Check sheet for the modelled part. Datum: model origin and axes. Units: mm. A direction names the side the tool comes from. Give positions to 0.01 mm unless a question says otherwise; leave off trailing zeros. Order: outer loops, then holes, each group sorted by start corner. A loop starts at its lowest first (then second) coordinate and runs counter-clockwise, first axis right, second up. Notation, with made-up numbers: (-5.5, 10.5) - (19.5, 10.5) arc R22 ccw to (19.5, 17.5) - close; hole circle Ø1 at (72, 24.25). An arc over 180 degrees is marked (long way). Answer in a Markdown table with one row per item.
from build123d import *

# Parameters (mm, degrees)
SKETCH1_R           = 10.5
BOSS_EXTRUDE1_DEPTH = 42
SKETCH3_R           = 14
BOSS_EXTRUDE2_DEPTH = 243
SKETCH4_R           = 9
BOSS_EXTRUDE3_DEPTH = 5
SKETCH5_W           = 36.2
SKETCH5_H           = 36.2
BOSS_EXTRUDE4_DEPTH = 35
BOSS_EXTRUDE4_TAPER = 5.710593137
SKETCH6_R           = 8
BOSS_EXTRUDE6_DEPTH = 3
SKETCH7_R           = 12
BOSS_EXTRUDE7_DEPTH = 25
CHAMFER1_SIZE       = 2
FILLET2_R           = 2.5
SKETCH8_W           = 3.5
SKETCH8_H           = 10
CHAMFER2_SIZE       = 2
CHAMFER3_SIZE       = 1
FILLET3_R           = 1.5


with BuildPart() as part:
    # Sketch1 → Boss-Extrude1 (new body)
    with BuildSketch(Plane(origin=(0, 0, 0), x_dir=(1, 0, 0), z_dir=(0, 1, 0))):
        with Locations(Location((0, 0, 0), (0, 0, 90))):
            Circle(SKETCH1_R)
    extrude(amount=BOSS_EXTRUDE1_DEPTH)

    # Sketch3 → Boss-Extrude2 (add)
    with BuildSketch(Plane(origin=(0, 42, 0), x_dir=(1, 0, 0), z_dir=(0, 1, 0))):
        with Locations(Location((0, 0, 0), (0, 0, 270))):
            Circle(SKETCH3_R)
    extrude(amount=BOSS_EXTRUDE2_DEPTH)

    # Sketch4 → Boss-Extrude3 (add)
    with BuildSketch(Plane(origin=(0, 285, 0), x_dir=(1, 0, 0), z_dir=(0, 1, 0))):
        with Locations(Location((0, 0, 0), (0, 0, 270))):
            Circle(SKETCH4_R)
    extrude(amount=BOSS_EXTRUDE3_DEPTH)

    # Sketch5 → Boss-Extrude4 (add)
    with BuildSketch(Plane(origin=(0, 290, 0), x_dir=(1, 0, 0), z_dir=(0, 1, 0))):
        Rectangle(SKETCH5_W, SKETCH5_H)
    extrude(amount=BOSS_EXTRUDE4_DEPTH, taper=BOSS_EXTRUDE4_TAPER)

    # Sketch6 → Boss-Extrude6 (add)
    with BuildSketch(Plane(origin=(0, 325, 0), x_dir=(1, 0, 0), z_dir=(0, 1, 0))):
        with Locations(Location((0, 0, 0), (0, 0, 270))):
            Circle(SKETCH6_R)
    extrude(amount=BOSS_EXTRUDE6_DEPTH)

    # Sketch7 → Boss-Extrude7 (add)
    with BuildSketch(Plane(origin=(0, 328, 0), x_dir=(1, 0, 0), z_dir=(0, 1, 0))):
        with Locations(Location((0, 0, 0), (0, 0, 270))):
            Circle(SKETCH7_R)
    extrude(amount=BOSS_EXTRUDE7_DEPTH)

    # Chamfer1
    chamfer1_edges = [part.edges().sort_by_distance(p)[0] for p in [
        (0, 328, -12),
        (0, 353, -12),
    ]]
    chamfer(chamfer1_edges, length=CHAMFER1_SIZE)

    # Fillet2
    fillet2_edges = [part.edges().sort_by_distance(p)[0] for p in [
        (0, 290, -9),
        (0, 285, -9),
    ]]
    fillet(fillet2_edges, radius=FILLET2_R - 0.0001)  # a hair under: the kernel refuses the full size

    # Sketch8 → Cut-Revolve1 (revolve, cut)
    with BuildSketch(Plane.XY, mode=Mode.PRIVATE) as cut_revolve1_sk:
        with Locations((-8.75, 20)):
            Rectangle(SKETCH8_W, SKETCH8_H)
    revolve(cut_revolve1_sk.sketch.rotate(Axis((0, 42, 0), (0, -1, 0)), 90), axis=Axis((0, 42, 0), (0, -1, 0)), mode=Mode.SUBTRACT)

    # Chamfer2
    chamfer2_edges = [part.edges().sort_by_distance(p)[0] for p in [
        (0, 42, -14),
        (0, 285, -14),
    ]]
    chamfer(chamfer2_edges, length=CHAMFER2_SIZE)

    # Chamfer3
    chamfer3_edges = [part.edges().sort_by_distance(p)[0] for p in [
        (0, 0, 10.5),
    ]]
    chamfer(chamfer3_edges, length=CHAMFER3_SIZE)

    # Fillet3
    fillet3_edges = [part.edges().sort_by_distance(p)[0] for p in [
        (0, 325, -8),
        (0, 328, -8),
    ]]
    fillet(fillet3_edges, radius=FILLET3_R - 0.0001)  # a hair under: the kernel refuses the full size


solid = part.part
(1) Cross-section at A-A, the plane y = 208. Record the cut outline in (x, z).
Geometry says:
| item | result |
|---|---|
| outline | circle Ø28 at (0, 0) |
(2) Access from +Z, -Z, +X, -X, +Y, -Y to the whole of each face (thin tool, end or side, straight path). Record for faces 1 (the flat face through (-11, 42, 0)), 2 (the flat face through (0, 0, 0)), 3 (the cylindrical face through (3.604, 340.353, 11.446)), 4 (the flat face through (-9, 290, -8)).
Geometry says:
| item | result |
|---|---|
| face 1 | -Y |
| face 2 | +Z, -Z, +X, -X, -Y |
| face 3 | +Y |
| face 4 | none |
(3) Thickness scan on L1, parallel to Y at x = -7, z = 3; L2, parallel to Y at x = -6.5, z = 8; L3, parallel to X at y = 227, z = -8. Record the ranges inside material, lowest first.
Geometry says:
| item | result |
|---|---|
| L1 | 0 to 15, 25 to 353 |
| L2 | 0.81 to 15, 25 to 285.3, 289.7 to 325, 328.31 to 352.69 |
| L3 | -11.49 to 11.49 |
(4) Gauge pin test, flat ends, axial feed: P1, Ø3, axis at x = 10, z = -1.5, coming from the +Y side; P2, Ø2, axis at x = -11, z = 2, coming from the -Y side; P3, Ø2, axis at y = 196.5, z = -4.5, coming from the +X side; P4, Ø1, axis at y = 186, z = 11.5, coming from the -X side. Record the tip position at first contact, or that the pin passes through.
Geometry says:
| item | result |
|---|---|
| P1 | y = 353 |
| P2 | y = 0.68 |
| P3 | x = 13.56 |
| P4 | x = -8.66 |
(5) Mould release check, pull along Y, two halves, no side actions. Record for faces 5 (the cylindrical face through (-3.2, 33.4, -10)), 6 (the flat face through (0, 353, 0)), 7 (the flat face through (-4, 328, 9)): pulls with the +Y half, pulls with the -Y half, needs draft (parallel to the pull), parting line crosses it, or undercut.
Geometry says:
| item | result |
|---|---|
| face 5 | needs draft |
| face 6 | pulls with the +Y half |
| face 7 | undercut |
